from build123d import *

# Parameters (mm, degrees)
F1_DEPTH = 304.8


with BuildPart() as f1:
    # F0 (on Right) → F1 (new body)
    with BuildSketch(Plane.YZ):
        with BuildLine():
            Line((-14.639986, 19.898164), (-16.386236, 19.898164))
            Line((-16.386236, 19.898164), (-16.386236, -17.408086))
            ThreePointArc((-16.386236, -17.408086), (-16.153752, -17.969352), (-15.592486, -18.201836))
            Line((-15.592486, -18.201836), (34.413764, -18.201836))
            Line((34.413764, -18.201836), (34.413764, -16.455586))
            ThreePointArc((34.413764, -16.455586), (34.18128, -15.89432), (33.620014, -15.661836))
            Line((33.620014, -15.661836), (-13.846236, -15.661836))
            Line((-13.846236, -15.661836), (-13.846236, 19.104414))
            ThreePointArc((-13.846236, 19.104414), (-14.07872, 19.66568), (-14.639986, 19.898164))
        make_face()
    extrude(amount=F1_DEPTH)


solid = f1.part
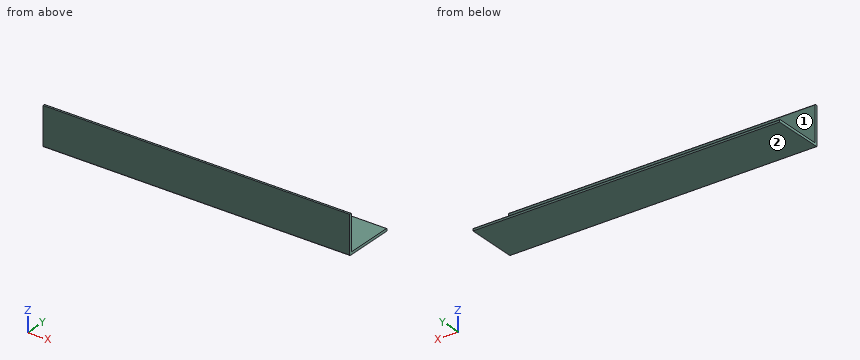
Verification items for the finished model (mm, model axes). Face numbers are marked on the shaded views. A direction names the side the tool comes from. Coordinates: 2 decimals unless noted, no trailing zeros. Write each loop counter-clockwise with the first axis right and the second up, starting at its lowest first coordinate (ties: lowest second). Pieces come first, ordered by that corner, then holes. Notation, with made-up numbers: (11, 20) -> (69, 20) arc R26 ccw to (69, 34) -> close; hole circle Ø3 at (82.25, 82). An arc over 180 degrees is marked (long way). One line per item, written item: value. Start each with the question number.
Q1. Cross-section at C-C on z = 1.5. Enter the section's corners in (x, y), and give its area (3 significant figures).
Q2. Cross-section at A-A on x = 28. Enter the section's corners in (y, z).
Q3. Cross-section at B-B on y = 11. Enter the section's corners in (x, z).
Q4. Go/stop test with flat-tipped pins: P1, Ø5, axis at x = 121, y = 27.5, coming from the +Z side; P2, Ø17.5, axis at x = 181.5, z = 3.5, coming from the +Y side. Record where each tip stops, or that it passes through.
Q5. Access from +Z, -Z, +X, -X, +Y, -Y to the whole of each face (thin tool, end or side, straight path). Record for the marked faces 1 and 2.
Q6. Thickness scan on L1, parallel to Z at x = 59, y = 20; L2, parallel to Y at x = 174, z = 14.5. Record the ranges inside material, lowest first. Write a range as from..to.
Checked values:
1. outline: (0, -16.39) -> (304.8, -16.39) -> (304.8, -13.85) -> (0, -13.85) -> close
1. area: 774 mm²
2. outline: (-16.39, -17.41) arc R0.79 ccw to (-15.59, -18.2) -> (34.41, -18.2) -> (34.41, -16.46) arc R0.79 ccw to (33.62, -15.66) -> (-13.85, -15.66) -> (-13.85, 19.1) arc R0.79 ccw to (-14.64, 19.9) -> (-16.39, 19.9) -> close
3. outline: (0, -18.2) -> (304.8, -18.2) -> (304.8, -15.66) -> (0, -15.66) -> close
4. P1: stops at z = -15.66
4. P2: stops at y = -13.85
5. face 1: +Z, +X, -X, +Y
5. face 2: -Z, +X, -X, +Y, -Y
6. L1: z = -18.2..-15.66
6. L2: y = -16.39..-13.85
